The listing builds one solid part. Answer for the finished solid, in the listing's coordinates (mm). Face numbers are marked on the shaded views. A direction names the side the tool comes from. Give positions to 0.01 mm unless a question says otherwise; leave off trailing zeros. Loops run counter-clockwise (first coordinate to the right, second up) from the corner with the lowest first, then second, coordinate; pieces in that order, holes last. Notation, with made-up numbers: M 0.25,-37.5 L 43.25,-37.5 A24 cw 43.25,-0.5 Z; hole C 48,32 d4. An arc over 180 degrees is marked long. Use one line per item in the form item = value. Start each with the question number.
1. The mould has two halves that part along X. Classify the marked faces 4, 5 and 6: released by +X, released by -X, zero draft, split by the parting line, or undercut.
2. The part is cut by section C-C (x = 17). Write down the section's boundary in (y, z), and give its area (3 significant figures).
3. The part is cut by section B-B (z = -5.75). Write down the section's boundary in (x, y).
4. Each of these flat-tipped pins is pushed along its axis until it touches: pin 1 Ø2 at (x, y) = (15.5, 16.5) entering from +Z; pin 2 Ø5 at (y, z) = (22.5, 0.5) entering from +X; pin 3 Ø3 at (x, z) = (20.5, 7) entering from +Y. Where does it stop, or does it pass through?
5. Straight lines are drawn through the part: line 1 (Z direction, x = 47.5, y = 3); line 2 (X direction, y = 10, z = 0); line 3 (Z direction, x = 36, y = 10.75). For each, find the intervals that lie inside material, in ascending order. Write a range as from..to.
6. The part is cut by section D-D (z = 12.25). Write down the section's boundary in (x, y).
7. The part is cut by section A-A (x = 36). Write down the section's boundary in (y, z).
8. For the marked faces 1, 2 and 3, determine the directions among +Z, -Z, +X, -X, +Y, -Y from which every point of the face is accessible in a straight line to the end or side of a thin tool.
Autodesk Fusion 360 part; units mm, degrees
sketch "Sketch1" plane through (0, 0, 0) normal (0, 0, 1) x (1, 0, 0)
  line L0 (0, 0) -> (0, 28)
  line L1 (0, 28) -> (14, 28)
  line L2 (14, 28) -> (14, 14)
  line L3 (14, 14) -> (50, 14)
  line L4 (50, 14) -> (50, 0)
  line L5 (50, 0) -> (0, 0)
  dimension "d1" = 14
  dimension "d2" = 14
  dimension "d3" = 14
  dimension "d4" = 50
extrude "Extrude1" add sketch "Sketch1" along normal mid plane 28
sketch "Sketch2" plane through (0, 0, 0) normal (0, 0, 1) x (1, 0, 0)
  line L0 (14, 28) -> (21, 28)
  line L1 (21, 28) -> (21, 14)
  line L2 (21, 14) -> (14, 14)
  line L3 (14, 14) -> (14, 28)
  point P0 (14, 28)
  point P1 (14, 14)
  dimension "d7" = 7
  dimension "d8" = 14
extrude "Extrude2" add sketch "Sketch2" against normal blind 14
sketch "Sketch3" plane through (50, 0, 0) normal (1, 0, 0) x (0, 0, -1)
  line L0 (14, 14) -> (-14, 14)
  line L1 (-14, 14) -> (-14, 0)
  line L2 (-14, 0) -> (14, 0)
  line L3 (14, 0) -> (14, 14)
  line L4 (-6.3263, 0) -> (-6.3263, 7)
  line L5 (-6.3263, 7) -> (7.6737, 7)
  line L6 (7.6737, 7) -> (7.6737, 0)
  line L7 (0, 18) -> (0, 0) construction
  line L8 (0, 0) -> (0, -4) construction
  dimension "d11" = 14
  dimension "d12" = 14
  dimension "d13" = 14
  dimension "d14" = 7.6737
  dimension "d15" = 90
  dimension "d16" = 7
extrude "Extrude3" cut sketch "Sketch3" against normal blind 50 contours L2 L4 L5 L6
sketch "Sketch4" plane through (0, 14, 0) normal (0, 1, 0) x (-1, 0, 0)
  line L0 (-21, -14) -> (-21, 0)
  line L1 (-21, 0) -> (-14, 0)
  line L2 (-14, 0) -> (-14, 14)
  line L3 (-14, 14) -> (-50, 14)
  line L4 (-50, 14) -> (-50, -14)
  line L5 (-50, -14) -> (-21, -14)
  line L6 (5.2801, -7) -> (-65, -7) construction
  line L7 (5, 7) -> (-62.1492, 7) construction
  circle A0 centre (-36, 0) radius 7
  dimension "d19" = 7
  dimension "d20" = 7
  dimension "d21" = 14
  dimension "d22" = 14
extrude "Extrude4" cut sketch "Sketch4" against normal blind 7 contours A0
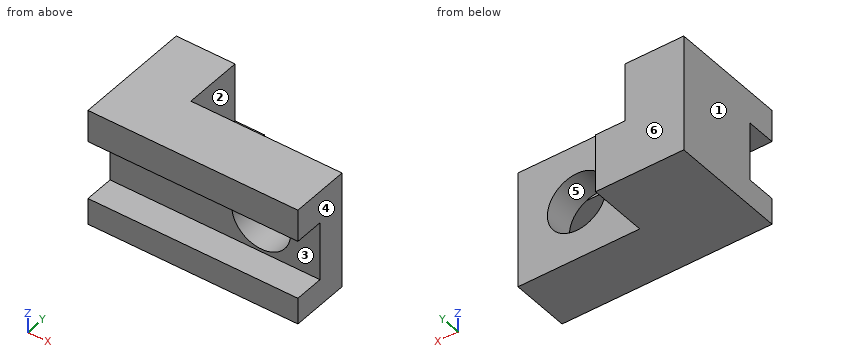
Derived:
q1.face_4 = released by +X
q1.face_5 = undercut
q1.face_6 = zero draft
q2.outline = M 0,-14 L 28,-14 L 28,0 L 14,0 L 14,14 L 0,14 L 0,6.33 L 7,6.33 L 7,-7.67 L 0,-7.67 Z
q2.area = 490 mm2
q3.outline = M 0,7 L 32.01,7 L 32.01,14 L 21,14 L 21,28 L 0,28 Z; M 39.99,7 L 50,7 L 50,14 L 39.99,14 Z
q4.pin_1 = 0
q4.pin_2 = 21
q4.pin_3 = 14
q5.line_1 = -14..-7.67, 6.33..14
q5.line_2 = 0..29, 43..50
q5.line_3 = -14..-7, 7..14
q6.outline = M 0,0 L 50,0 L 50,14 L 14,14 L 14,28 L 0,28 Z
q7.outline = M 0,-14 L 14,-14 L 14,-7 L 7,-7 L 7,-7.67 L 0,-7.67 Z; M 0,6.33 L 7,6.33 L 7,7 L 14,7 L 14,14 L 0,14 Z
q8.face_1 = +Z, -Z, -X, +Y, -Y
q8.face_2 = +Z, +X, +Y
q8.face_3 = +X, -X, -Y
